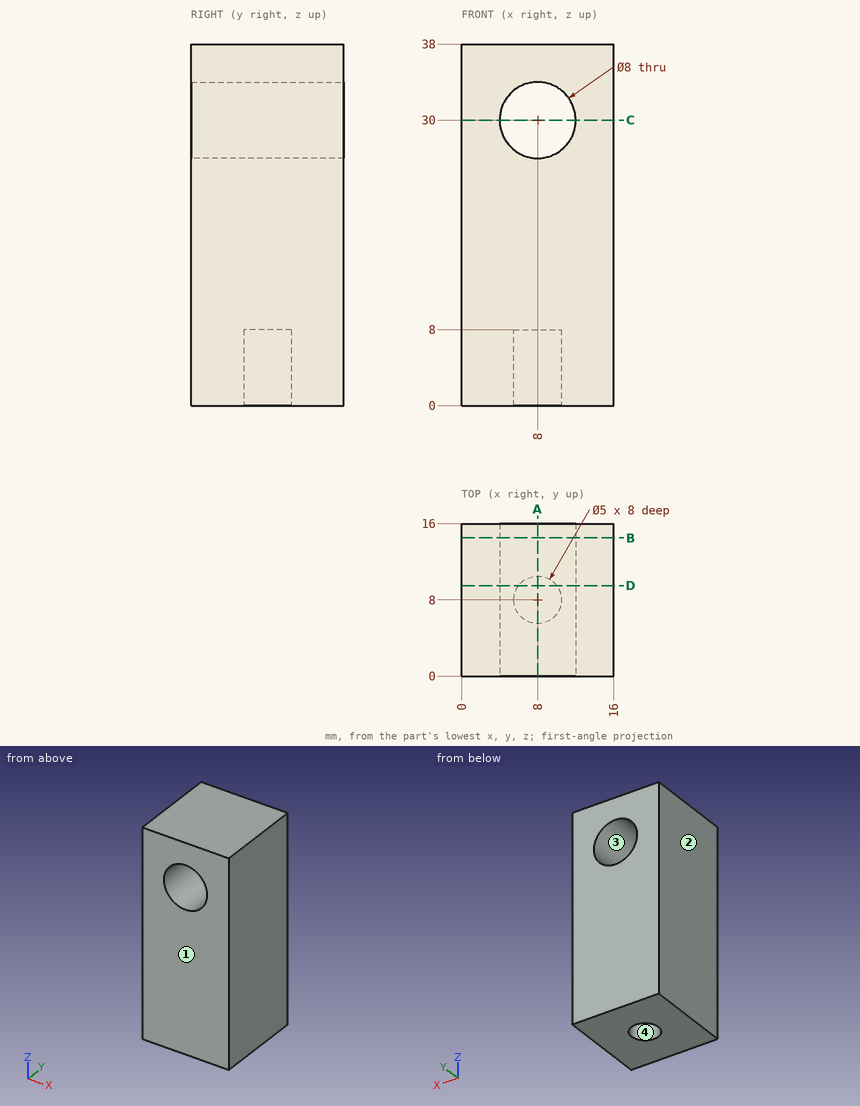
Geometry: see drawing. Coordinates: mm, zero at the bounding-box minimum. Round coordinates to 2 decimals unless told otherwise and drop trailing zeros. Order: outer loops, then holes, each group sorted by start corner. A loop starts at its lowest first (then second) coordinate and runs counter-clockwise, first axis right, second up. Notation, with made-up numbers: (46.25, -36.75) -> (67.25, -36.75) arc R21 cw to (67.25, -17.75) -> close; hole circle Ø7 at (-28, 22). An arc over 180 degrees is marked (long way). Write each question's results on one line, items separated by ' | '.
Q1. Section query C-C (z = 30). Output: boundary loops of the cut face in (x, y), and give its area (3 significant figures).
Response values:
outline: (0, 0) -> (4, 0) -> (4, 16) -> (0, 16) -> close; (12, 0) -> (16, 0) -> (16, 16) -> (12, 16) -> close | area: 128 mm²
Q2. Section query A-A (x = 8). Output: boundary loops of the cut face in (y, z).
Response values:
outline: (0, 0) -> (5.5, 0) -> (5.5, 8) -> (10.5, 8) -> (10.5, 0) -> (16, 0) -> (16, 26) -> (0, 26) -> close; (0, 34) -> (16, 34) -> (16, 38) -> (0, 38) -> close
Q3. Pull-direction query (X, two-part tool) for the marked faces 1, 2, 3 and 4; classes: released by +X, released by -X, zero draft, split by the parting line, or undercut.
Response values:
face 1: zero draft | face 2: released by -X | face 3: undercut | face 4: undercut
Q4. Ray query, line 1 along Y through (x, z) = (8, 3); line 2 along Z through (x, y) = (7.75, 6.5); line 3 along X through (y, z) = (4.5, 30). Return the intervals inside material, ascending.
Response values:
line 1: 0 to 5.5, 10.5 to 16 | line 2: 8 to 26.01, 33.99 to 38 | line 3: 0 to 4, 12 to 16
Q5. Section query D-D (y = 9.5). Output: boundary loops of the cut face in (x, z).
Response values:
outline: (0, 0) -> (6, 0) -> (6, 8) -> (10, 8) -> (10, 0) -> (16, 0) -> (16, 38) -> (0, 38) -> close; hole circle Ø8 at (8, 30)
Q6. Section query B-B (y = 14.5). Output: boundary loops of the cut face in (x, z).
Response values:
outline: (0, 0) -> (16, 0) -> (16, 38) -> (0, 38) -> close; hole circle Ø8 at (8, 30)
